Source: CAD feature listing. Evaluate the final solid. Frame: model axes, mm. A direction names the side the tool comes from. Round coordinates to 2 decimals unless told otherwise and drop trailing zeros. Order: outer loops, then holes, each group sorted by start corner. A loop starts at its lowest first (then second) coordinate and runs counter-clockwise, first axis right, second up. Notation, with made-up numbers: (15.25, 15.5) - (57.25, 15.5) arc R17 ccw to (57.25, 33.5) - close; hole circle Ø8 at (69.25, 71). An arc over 180 degrees is marked (long way). Return JSON: item names as keys, results as strings. Group by question number.
1) Section C-C, the plane y = 0. Give the number of separate pieces and of enclosed holes in the cut face, plus the area to 3 significant figures.
2) Section B-B, the plane z = 10. Return loops of the section in (x, y).
3) Contact query for flat-ended pins moving along their axis: P1, Ø1, axis at y = 9.5, z = 2.5, coming from the -X side; P2, Ø1.5, axis at x = -10, y = 0, coming from the +Z side; P3, Ø2.5, axis at y = -8.66, z = -5, coming from the -X side. Output: stop coordinate, or through.
4) Section A-A, the plane z = -5. Return loops of the section in (x, y), plus the area to 3 significant figures.
5) Access query for faces 1 (the flat face through (-4, 0, -1.2)), 2 (the flat face through (-12, -2, 2)), 3 (the cylindrical face through (0.99, 1.43, -2.75)). Directions: +Z, -Z, +X, -X, +Y, -Y. A direction counts if a zero-diameter tool reaches every point of the face in a straight line with its end or side. Return the directions, or none.
6) Section D-D, the plane y = -5. Return loops of the section in (x, z).
7) Ray query, line 1 (Z direction, x = 0.25, y = 0); line 2 (Z direction, x = -0.35, y = 0); line 3 (X direction, y = 1, z = -9). Return the intervals inside material, ascending. Write a range as from..to.
8) Mould query, pull axis Z, two halves, no side actions, for faces 4 (the flat face through (1, 9.5, -5.8)), 5 (the flat face through (-1, -1, 9)), 6 (the cylindrical face through (0.493, 9.682, -3.398)). Classes: pulls with the +Z half, pulls with the -Z half, needs draft (parallel to the pull), parting line crosses it, or undercut.
```python
from build123d import *

# Parameters (mm, degrees)
F0_R      = 13
F0_R_2    = 1
F0_R_3    = 2
F1_DEPTH  = 2
F4_R      = 4
F4_R_2    = 1
F5_DEPTH  = 10
F6_R      = 2.5
F6_R_2    = 1
F7_DEPTH  = 1
F8_R      = 1
F9_DEPTH  = 8
F2_R      = 1.9
F2_R_2    = 1
F10_DEPTH = 1
F3_R      = 3.1
F3_R_2    = 2
F11_DEPTH = 2


with BuildPart() as f1:
    # F0 (on Right) → F1 (new body)
    with BuildSketch(Plane.YZ):
        Circle(F0_R)
        with Locations((-8.660254, -5)):
            Circle(F0_R_2, mode=Mode.SUBTRACT)
        with Locations((8.660254, -5)):
            Circle(F0_R_2, mode=Mode.SUBTRACT)
        Circle(F0_R_3, mode=Mode.SUBTRACT)
        with Locations((0, 10)):
            Circle(F0_R_2, mode=Mode.SUBTRACT)
    extrude(amount=-F1_DEPTH)

    # F4 (on face) → F5 (join)
    with BuildSketch(Plane(origin=(-2, 0, 0), x_dir=(0, -1, 0), z_dir=(-1, 0, 0))):
        Circle(F4_R)
        Circle(F4_R_2, mode=Mode.SUBTRACT)
    extrude(amount=F5_DEPTH)

    # F6 (on face) → F7 (cut)
    with BuildSketch(Plane(origin=(-2, 0, 0), x_dir=(0, -1, 0), z_dir=(-1, 0, 0))):
        with Locations((0, 10)):
            Circle(F6_R)
        with Locations((0, 10)):
            Circle(F6_R_2, mode=Mode.SUBTRACT)
        with Locations((8.660254, -5)):
            Circle(F6_R)
        with Locations((8.660254, -5)):
            Circle(F6_R_2, mode=Mode.SUBTRACT)
        with Locations((-8.660254, -5)):
            Circle(F6_R)
        with Locations((-8.660254, -5)):
            Circle(F6_R_2, mode=Mode.SUBTRACT)
    extrude(amount=-F7_DEPTH, mode=Mode.SUBTRACT)

    # F8 (on face) → F9 (cut)
    with BuildSketch(Plane(origin=(-12, 0, 0), x_dir=(0, -1, 0), z_dir=(-1, 0, 0))):
        Circle(F8_R)
        with BuildLine():
            ThreePointArc((-1.5, 2), (-1.118034, -2.236068), (2.5, 0))
            ThreePointArc((2.5, 0), (2.236068, 1.118034), (1.5, 2))
            Line((1.5, 2), (-1.5, 2))
        make_face()
        Circle(F8_R, mode=Mode.SUBTRACT)
    extrude(amount=-F9_DEPTH, mode=Mode.SUBTRACT)

    # F2 (on face) → F10 (join)
    with BuildSketch(Plane.YZ):
        with Locations((0, 10)):
            Circle(F2_R)
        with Locations((0, 10)):
            Circle(F2_R_2, mode=Mode.SUBTRACT)
        with Locations((8.660254, -5)):
            Circle(F2_R)
        with Locations((8.660254, -5)):
            Circle(F2_R_2, mode=Mode.SUBTRACT)
        with Locations((-8.660254, -5)):
            Circle(F2_R)
        with Locations((-8.660254, -5)):
            Circle(F2_R_2, mode=Mode.SUBTRACT)
    extrude(amount=F10_DEPTH)

    # F3 (on face) → F11 (join)
    with BuildSketch(Plane.YZ):
        Circle(F3_R)
        Circle(F3_R_2, mode=Mode.SUBTRACT)
    extrude(amount=F11_DEPTH)


solid = f1.part
```
Geometry check:
{
 "1": {"separate pieces": "3", "enclosed holes": "0", "area": "83.2 mm2"},
 "2": {"outline": "(-2, -8.31) - (0, -8.31) - (0, -1.9) - (1, -1.9) - (1, -1) - (-1, -1) - (-1, -2.5) - (-2, -2.5) - close; (-2, 2.5) - (-1, 2.5) - (-1, 1) - (1, 1) - (1, 1.9) - (0, 1.9) - (0, 8.31) - (-2, 8.31) - close"},
 "3": {"P1": "x = -2", "P2": "z = 4", "P3": "x = -1"},
 "4": {"outline": "(-2, -12) - (0, -12) - (0, -10.56) - (1, -10.56) - (1, -9.66) - (-1, -9.66) - (-1, -11.16) - (-2, -11.16) - close; (-2, -6.16) - (-1, -6.16) - (-1, -7.66) - (1, -7.66) - (1, -6.76) - (0, -6.76) - (0, 6.76) - (1, 6.76) - (1, 7.66) - (-1, 7.66) - (-1, 6.16) - (-2, 6.16) - close; (-2, 11.16) - (-1, 11.16) - (-1, 9.66) - (1, 9.66) - (1, 10.56) - (0, 10.56) - (0, 12) - (-2, 12) - close", "area": "37.6 mm2"},
 "5": {"face 1": "-X", "face 2": "+Z, -Z, -X, +Y, -Y", "face 3": "+X"},
 "6": {"outline": "(-2, -12) - (0, -12) - (0, 12) - (-2, 12) - close"},
 "7": {"line 1": "-3.1..-2, 2..3.1, 8.1..9, 11..11.9", "line 2": "-13..-2, 2..9, 11..13", "line 3": "-2..0"},
 "8": {"face 4": "needs draft", "face 5": "undercut", "face 6": "parting line crosses it"}
}
